For this review, take the finished solid that the model builds, in its own axes (mm). Give positions to 0.01 mm unless a question says otherwise; leave off trailing zeros. Order: outer loops, then holes, each group sorted by start corner. A loop starts at its lowest first (then second) coordinate and runs counter-clockwise, first axis right, second up. Notation, with made-up numbers: (70, 40.25) -> (85, 40.25) arc R26 cw to (85, 77.25) -> close; hole circle Ø11 at (25.25, -27.75). An arc over 180 degrees is marked (long way). One line per item, written item: value. Start each with the question number.
from build123d import *

# Parameters (mm, degrees)
F0_W           = 266.7
F0_H           = 228.6
F1_DEPTH       = 3.175
F2_R           = 50.8
F4_D           = 4.9784
F4_CSINK_D     = 9.1186
F4_CSINK_ANGLE = 82
F5_R           = 38.1
F6_DEPTH       = 3.176


with BuildPart() as f1:
    # F0 (on Top) → F1 (new body)
    with BuildSketch(Plane.XY):
        Rectangle(F0_W, F0_H)
    extrude(amount=F1_DEPTH)

    # F2
    f2_edges = [f1.edges().sort_by_distance(p)[0] for p in [
        (-133.35, 114.3, 1.5875),
        (133.35, 114.3, 1.5875),
        (133.35, -114.3, 1.5875),
        (-133.35, -114.3, 1.5875),
    ]]
    fillet(f2_edges, radius=F2_R)

    # F4 (through all)
    with Locations(Plane(origin=(0, 0, 0), x_dir=(1, 0, 0), z_dir=(0, 0, -1))):
        with Locations((-127, -12.7), (-101.6, -12.7), (-101.6, 25.4), (-127, 25.4), (-127, 63.5), (-101.6, 63.5)):
            CounterSinkHole(F4_D / 2, F4_CSINK_D / 2, counter_sink_angle=F4_CSINK_ANGLE)

    # F5 (on face) → F6 (cut, through all)
    with BuildSketch(Plane.XY.offset(3.175)):
        with Locations((-31.75, 50.8)):
            Circle(F5_R)
        with Locations((69.85, 50.8)):
            Circle(F5_R)
        with Locations((-31.75, -50.8)):
            Circle(F5_R)
        with Locations((69.85, -50.8)):
            Circle(F5_R)
    extrude(amount=-F6_DEPTH, mode=Mode.SUBTRACT)


solid = f1.part
Q1. Take a section at B-B (y = 50.8). State the section outline as (x, z) points (3 decimals).
Q2. For pin 1 Ø5 at (x, y) = (19.5, -53.5) entering from -Z; pin 2 Ø5.5 at (x, y) = (-127, -63.5) entering from -Z, all flat-tipped, find the tip position at first contact; note any pin that passes through.
Q3. Take a section at A-A (x = -31.75). State the section outline as (y, z) points (3 decimals).
Q4. Mouldability with a two-part tool opening along X and no side actions: class faces 1 (the conical face through (-99.013, -25.514, 2.266)), 2 (the cylindrical face through (118.864, 99.024, 1.61)), 3 (the flat face through (-2, 2, 0)), 4 (the conical face through (-129.47, -64.278, 2.266)) as pulls with the +X half, pulls with the -X half, needs draft (parallel to the pull), parting line crosses it, or undercut.
Q5. Take a section at C-C (z = 0.7). State how many separate pieces and enclosed holes the cut face has, and give its area (3 significant figures).
Q6. For line 1 along Y through (x, z) = (69.85, 1.3); line 2 along X through (y, z) = (52, 1.2); line 3 along Y through (x, z) = (-101.6, 2.95), list the stretches that pass through material, from the lowest coordinate up.
Answers below:
1. outline: (-133.35, 0) -> (-69.85, 0) -> (-69.85, 3.175) -> (-133.35, 3.175) -> close; (6.35, 0) -> (31.75, 0) -> (31.75, 3.175) -> (6.35, 3.175) -> close; (107.95, 0) -> (133.35, 0) -> (133.35, 3.175) -> (107.95, 3.175) -> close
2. pin 1: stops at z = 0
2. pin 2: stops at z = 2.08
3. outline: (-114.3, 0) -> (-88.9, 0) -> (-88.9, 3.175) -> (-114.3, 3.175) -> close; (-12.7, 0) -> (12.7, 0) -> (12.7, 3.175) -> (-12.7, 3.175) -> close; (88.9, 0) -> (114.3, 0) -> (114.3, 3.175) -> (88.9, 3.175) -> close
4. face 1: undercut
4. face 2: pulls with the +X half
4. face 3: needs draft
4. face 4: undercut
5. separate pieces: 1
5. enclosed holes: 10
5. area: 40,200 mm²
6. line 1: y = -114.3 to -88.9, -12.7 to 12.7, 88.9 to 114.3
6. line 2: x = -133.35 to -69.83, 6.33 to 31.77, 107.93 to 133.35
6. line 3: y = -110.59 to -65.99, -61.01 to -27.89, -22.91 to 10.21, 15.19 to 110.59
